For this review, use the dimensioned drawing (mm, ordinates from the lowest corner) and the shaded views. A direction names the side the tool comes from. Coordinates: 2 decimals unless noted, no trailing zeros. Order: outer loops, then holes, each group sorted by start corner. A loop starts at its lowest first (then second) coordinate and runs counter-clockwise, first axis right, second up. Notation, with made-up numbers: M -31.5,3 L 27.5,3 A11 cw 27.5,17 Z; hole C 28,42.25 d3. An arc over 180 degrees is marked long. Answer as CSV lines item,"result". Start each with the question number.
Q1. Machinability: for the marked faces 4 and 5, which of the approach directions +Z, -Z, +X, -X, +Y, -Y give a long, thin tool a straight path to every point of the face, cutting with its end or side? Answer none if there is none.
Q2. For P1, Ø1, axis at x = 10.5, z = 7, coming from the +Y side; P2, Ø2, axis at x = 5, y = 3, coming from the -Z side, all flat-tipped, find the tip position at first contact; note any pin that passes through.
Q3. Consider section C-C on y = 1.3. Write out the cut boundary in (x, z), and give its area (3 significant figures).
Q4. Wall thickness on L1, parallel to Z at x = 6.75, y = 4.75; L2, parallel to Z at x = 6.75, y = 2.25; L3, parallel to Y at x = 5, z = 4: over which ranges is each line inside the solid? List them lowest first. Write a range as [from, to].
Q5. Consider section B-B on x = 6.75. Write out the cut boundary in (y, z) (3 decimals), and give its area (3 significant figures).
Q6. Consider section A-A on z = 6.75. Write out the cut boundary in (x, y) (3 decimals).
Q7. The part is to be moulded in two halves that separate along Z. For the marked faces 1, 2 and 3, say which applies: +Z half, -Z half, draft (parallel to the pull), parting line (faces both ways), or undercut.
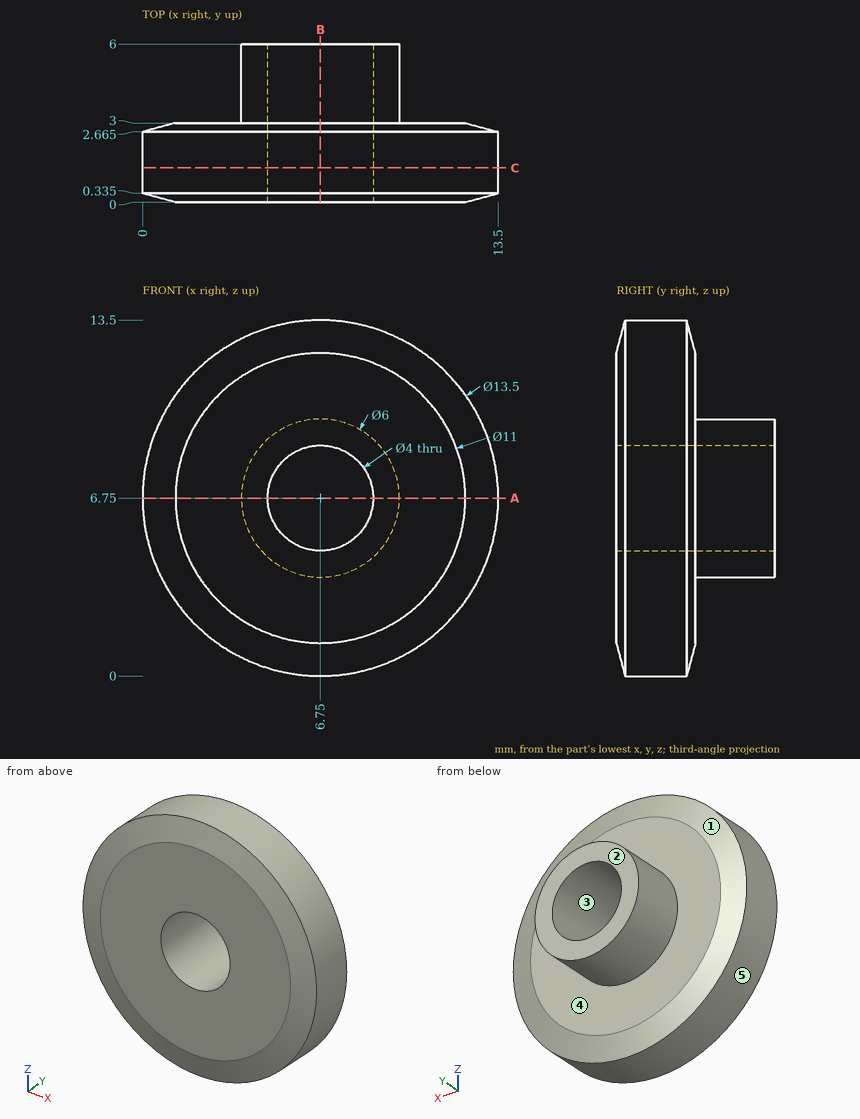
Evaluation:
1,face 4,"+Y"
1,face 5,"+Y, -Y"
2,P1,"stops at y = 3"
2,P2,"stops at z = 0.05"
3,outline,"C 6.75,6.75 d13.5; hole C 6.75,6.75 d4"
3,area,"131 mm²"
4,L1,"z = [3.75, 4.75], [8.75, 9.75]"
4,L2,"z = [0, 4.75], [8.75, 13.5]"
4,L3,"y = [0, 3]"
5,outline,"M 0,1.25 L 0.335,0 L 2.665,0 L 3,1.25 L 3,3.75 L 6,3.75 L 6,4.75 L 0,4.75 Z; M 0,8.75 L 6,8.75 L 6,9.75 L 3,9.75 L 3,12.25 L 2.665,13.5 L 0.335,13.5 L 0,12.25 Z"
5,area,"33.7 mm²"
6,outline,"M 0,0.335 L 1.25,0 L 4.75,0 L 4.75,6 L 3.75,6 L 3.75,3 L 1.25,3 L 0,2.665 Z; M 8.75,0 L 12.25,0 L 13.5,0.335 L 13.5,2.665 L 12.25,3 L 9.75,3 L 9.75,6 L 8.75,6 Z"
7,face 1,"parting line"
7,face 2,"draft"
7,face 3,"undercut"
